Autodesk Inventor part; units mm, degrees
ref_plane "Work Plane1" through (0, 0, 35.56) normal (0, 0, 1) x (1, 0, 0)
ref_plane "YZ Plane" through (0, 0, 0) normal (1, 0, 0) x (0, 1, 0)
ref_plane "XZ Plane" through (0, 0, 0) normal (0, 1, 0) x (-1, 0, 0)
sketch "Sketch1" plane through (0, 0, 0) normal (0, 0, 1) x (1, 0, 0)
  circle A0 centre (0, 0) radius 50.8
  dimension "d0" = 101.6
extrude "Extrusion1" add sketch "Sketch1" along normal blind 2.54
sketch "Sketch2" plane through (0, 0, 2.54) normal (0, 0, 1) x (1, 0, 0)
  circle A0 centre (0, 0) radius 50.8
  arc A1 (5.858, 50.4611) -> (-0.0279, 50.8) centre (0, 0) ccw
  arc A2 (12.9209, 13.9983) -> (9.6237, 16.4404) centre (0, 0) ccw
  line L0 (-0.0279, 50.8) -> (9.6237, 16.4404)
  line L1 (5.858, 50.4611) -> (12.9209, 13.9983)
  arc A3 (39.8236, 31.5392) -> (35.9013, 35.9408) centre (0, 0) ccw
  arc A4 (19.0348, 0.7618) -> (18.4301, 4.8202) centre (0, 0) ccw
  line L2 (35.9013, 35.9408) -> (18.4301, 4.8202)
  line L3 (39.8236, 31.5392) -> (19.0348, 0.7618)
  arc A5 (50.4611, -5.858) -> (50.8, 0.0279) centre (0, 0) ccw
  arc A6 (13.9983, -12.9209) -> (16.4404, -9.6237) centre (0, 0) ccw
  line L4 (50.8, 0.0279) -> (16.4404, -9.6237)
  line L5 (50.4611, -5.858) -> (13.9983, -12.9209)
  arc A7 (31.5392, -39.8236) -> (35.9408, -35.9013) centre (0, 0) ccw
  arc A8 (0.7618, -19.0348) -> (4.8202, -18.4301) centre (0, 0) ccw
  line L6 (35.9408, -35.9013) -> (4.8202, -18.4301)
  line L7 (31.5392, -39.8236) -> (0.7618, -19.0348)
  arc A9 (-5.858, -50.4611) -> (0.0279, -50.8) centre (0, 0) ccw
  arc A10 (-12.9209, -13.9983) -> (-9.6237, -16.4404) centre (0, 0) ccw
  line L8 (0.0279, -50.8) -> (-9.6237, -16.4404)
  line L9 (-5.858, -50.4611) -> (-12.9209, -13.9983)
  arc A11 (-39.8236, -31.5392) -> (-35.9013, -35.9408) centre (0, 0) ccw
  arc A12 (-19.0348, -0.7618) -> (-18.4301, -4.8202) centre (0, 0) ccw
  line L10 (-35.9013, -35.9408) -> (-18.4301, -4.8202)
  line L11 (-39.8236, -31.5392) -> (-19.0348, -0.7618)
  arc A13 (-50.4611, 5.858) -> (-50.8, -0.0279) centre (0, 0) ccw
  arc A14 (-13.9983, 12.9209) -> (-16.4404, 9.6237) centre (0, 0) ccw
  line L12 (-50.8, -0.0279) -> (-16.4404, 9.6237)
  line L13 (-50.4611, 5.858) -> (-13.9983, 12.9209)
  arc A15 (-31.5392, 39.8236) -> (-35.9408, 35.9013) centre (0, 0) ccw
  arc A16 (-0.7618, 19.0348) -> (-4.8202, 18.4301) centre (0, 0) ccw
  line L14 (-35.9408, 35.9013) -> (-4.8202, 18.4301)
  line L15 (-31.5392, 39.8236) -> (-0.7618, 19.0348)
  dimension "d7" = 360
extrude "Extrusion2" add sketch "Sketch2" along normal blind 30.48 contours A0 L5 A6 L4 | L3 A4 L2 A0 | A0 L7 A8 L6 | L1 A2 L0 A0 | A0 L9 A10 L8 | L15 A16 L14 A0 | A0 L11 A12 L10 | L13 A14 L12 A0
ref_plane "Work Plane1" through (0, 0, 35.56) normal (0, 0, 1) x (1, 0, 0)
sketch "Sketch3" plane through (0, 0, 35.56) normal (0, 0, 1) x (1, 0, 0)
  circle A0 centre (0, 0) radius 50.8
  dimension "d12" = 101.6
extrude "Extrusion3" add sketch "Sketch3" against normal blind 2.54
properties part number "Box fan"
Work out the finished part from the listing and answer in its coordinate system (mm). A direction names the side the tool comes from. Give positions to 0.01 mm unless a question says otherwise; leave off trailing zeros. Loops run counter-clockwise (first coordinate to the right, second up) from the corner with the lowest first, then second, coordinate; pieces in that order, holes last. Notation, with made-up numbers: (40.25, 42) -> (97.25, 42) arc R17 ccw to (97.25, 75) -> close; hole circle Ø3 at (84.25, 62.5). An arc over 180 degrees is marked (long way). Write item = value, one per line. Start each with the question number.
(1) Find section D-D on x = -30. Give the vertices of the cut face in (y, z), and give its area (3 significant figures).
(2) Find section B-B on z = 29. Give the number of separate pieces and of enclosed holes in the cut face, and give its area (3 significant figures).
(3) Find the intervals of material crossed by probe 1 along Z at (x, y) = (16.5, 33); probe 2 along X at (y, z) = (34, 16); probe 3 along X at (y, z) = (-32.5, 22.5), in increasing order. Write a range as from..to.
(4) Find section A-A on y = 20.5. Give the vertices of the cut face in (x, z).
(5) Find section C-C on x = -44. Give the vertices of the cut face in (y, z).
(6) Given pin 1 Ø2 at (x, z) = (1.5, 30) entering from +Y; pin 2 Ø6 at (x, z) = (-5, 21) entering from -Y; pin 3 Ø4 at (y, z) = (-10.5, 13) entering from -X, each flat-ended and moving along its own axis, determine where each tip first touches the part or whether it passes through.
(7) Which of the six approach directions +Z, -Z, +X, -X, +Y, -Y give full straight-line access (tool end or side, diameter ignored) to faces 5 (the cylindrical face through (-2.836, 18.838, 17.567)), 6 (the flat face through (-16.4, 29.6, 17.6)), 7 (the cylindrical face through (-15.325, 11.315, 17.567)), 8 (the flat face through (-32.48, 9.34, 17.57))?
(8) The mould has two halves that part along Z. Classify faces 1 (the flat face through (-1, 1, 0)), 2 (the flat face through (-1, 1, 35.56)), 3 (the flat face through (33.86, -4.73, 17.57)), 4 (the flat face through (-1, 1, 2.54)): +Z half, -Z half, draft (parallel to the pull), parting line (faces both ways), or undercut.
From the geometry:
q1.outline = (-41, 0) -> (41, 0) -> (41, 2.54) -> (38.78, 2.54) -> (38.78, 33.02) -> (41, 33.02) -> (41, 35.56) -> (-41, 35.56) -> (-41, 33.02) -> (-25.43, 33.02) -> (-25.43, 2.54) -> (-41, 2.54) -> close; hole (-17, 2.54) -> (5.81, 2.54) -> (5.81, 33.02) -> (-17, 33.02) -> close; hole (9.82, 2.54) -> (32.57, 2.54) -> (32.57, 33.02) -> (9.82, 33.02) -> close
q1.area = 985 mm^2
q2.separate_pieces = 8
q2.enclosed_holes = 0
q2.area = 1,210 mm^2
q3.probe_1 = 0..2.54, 33.02..35.56
q3.probe_2 = -32.55..-22.92, 4.69..9.05, 34.81..37.74
q3.probe_3 = -39.04..-33.97, -9.34..-5.11, 20.7..29.88
q4.outline = (-46.48, 0) -> (46.48, 0) -> (46.48, 2.54) -> (32.37, 2.54) -> (32.37, 33.02) -> (46.48, 33.02) -> (46.48, 35.56) -> (-46.48, 35.56) -> (-46.48, 33.02) -> (-8.51, 33.02) -> (-8.51, 2.54) -> (-46.48, 2.54) -> close; hole (-2.93, 2.54) -> (8.48, 2.54) -> (8.48, 33.02) -> (-2.93, 33.02) -> close; hole (11.66, 2.54) -> (27.23, 2.54) -> (27.23, 33.02) -> (11.66, 33.02) -> close
q5.outline = (-25.39, 0) -> (25.39, 0) -> (25.39, 2.54) -> (7.11, 2.54) -> (7.11, 33.02) -> (25.39, 33.02) -> (25.39, 35.56) -> (-25.39, 35.56) -> (-25.39, 33.02) -> (1.88, 33.02) -> (1.88, 2.54) -> (-25.39, 2.54) -> close
q6.pin_1 = 50.8
q6.pin_2 = -50.76
q6.pin_3 = -26.96
q7.face_5 = none
q7.face_6 = +Y
q7.face_7 = -Y
q7.face_8 = -X
q8.face_1 = -Z half
q8.face_2 = +Z half
q8.face_3 = undercut
q8.face_4 = undercut
